Design review of the part shown in the three views and the two pictorial views. Dimensions are in mm from the part's minimum x, y and z. A direction names the side the tool comes from. Coordinates: 2 decimals unless noted, no trailing zeros. Order: outer loops, then holes, each group sorted by start corner. A loop starts at its lowest first (then second) coordinate and runs counter-clockwise, first axis right, second up. Notation, with made-up numbers: M 59.5,-11 L 118.5,-11 A15 cw 118.5,1 Z; hole C -36,-5.5 d4. An arc over 180 degrees is marked long. Use CSV: the item, a comma, the result in double quotes.
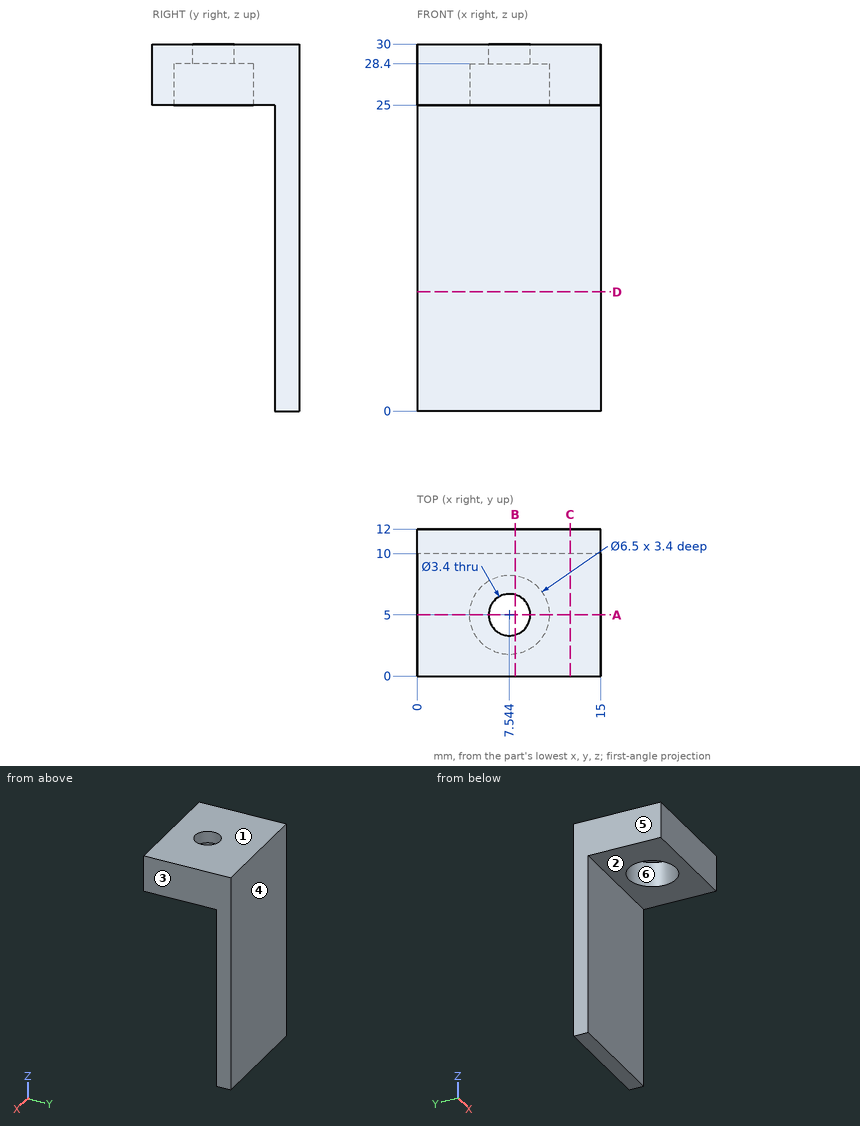
(1) Add section B-B on x = 8. State the section outline as (y, z) points.
The answers:
outline,"M 0,25 L 1.78,25 L 1.78,28.4 L 3.36,28.4 L 3.36,30 L 0,30 Z; M 6.64,28.4 L 8.22,28.4 L 8.22,25 L 10,25 L 10,0 L 12,0 L 12,30 L 6.64,30 Z"
(2) Add section C-C on x = 12.5. State the section outline as (y, z) points.
The answers:
outline,"M 0,25 L 10,25 L 10,0 L 12,0 L 12,30 L 0,30 Z"
(3) Add section A-A on y = 5. State the section outline as (x, z) points.
The answers:
outline,"M 0,25 L 4.29,25 L 4.29,28.4 L 5.84,28.4 L 5.84,30 L 0,30 Z; M 9.24,28.4 L 10.79,28.4 L 10.79,25 L 15,25 L 15,30 L 9.24,30 Z"
(4) Clearance check with flat-ended pins moving along their axes: P1, Ø4, axis at x = 9, y = 1.5, coming from the -Z side; P2, Ø4.5, axis at x = 5.5, z = 11, coming from the -Y side; P3, Ø3, axis at x = 7, y = 6, coming from the -Z side. State where each tip first meets the part, or that it passes through.
The answers:
P1,"stops at z = 25"
P2,"stops at y = 10"
P3,"stops at z = 28.4"
(5) For the marked faces 1 and 2, list the 3-axis set-ups (+Z, -Z, +X, -X, +Y, -Y) from which the entire face can be reached by the end or side of a thin tool; tool diameter is ignored.
The answers:
face 1,"+Z, +X, -X, +Y, -Y"
face 2,"-Z, +X, -X, -Y"
(6) Wall thickness on probe 1 along Y at (x, z) = (9.25, 8); probe 2 along Z at (x, y) = (7, 1); probe 3 along Z at (x, y) = (6, 7.25): over which ranges is each line inside the solid? List them lowest first.
The answers:
probe 1,"y = 10 to 12"
probe 2,"z = 25 to 30"
probe 3,"z = 28.4 to 30"
(7) The part is to be moulded in two halves that separate along X. For the marked faces 3, 4, 5 and 6, say which applies: pulls with the +X half, pulls with the -X half, needs draft (parallel to the pull), parting line crosses it, or undercut.
The answers:
face 3,"pulls with the +X half"
face 4,"needs draft"
face 5,"pulls with the -X half"
face 6,"undercut"
(8) Add section D-D on z = 9.75. State the section outline as (x, y) points, and give its area (3 significant figures).
The answers:
outline,"M 0,10 L 15,10 L 15,12 L 0,12 Z"
area,"30.0 mm2"
